For this review, take the finished solid that the model builds, in its own axes (mm). A direction names the side the tool comes from. Coordinates: 2 decimals unless noted, no trailing zeros. Order: outer loops, then holes, each group sorted by start corner. A loop starts at its lowest first (then second) coordinate and runs counter-clockwise, first axis right, second up. Notation, with made-up numbers: (-34.5, 6) -> (-6.5, 6) arc R17 ccw to (-6.5, 31) -> close; hole circle Ø11 at (38.25, -38). An arc over 180 degrees is marked (long way). Write item = value, one per line. Start each with the question number.
1) Insertion check: pin 1 Ø4.5 at (x, z) = (77, 50.13) entering from -Y; pin 2 Ø2 at (y, z) = (1, -73.5) entering from -X; pin 3 Ø1.1 at (y, z) = (4.5, -68) entering from -X; pin 4 Ø3 at (y, z) = (1, 76) entering from -X. Each pin has a flat end and moves straight along its axis. Give the tip position at first contact, or say it passes through.
2) Consider section D-D on x = 22. Give the boundary of the cut face in (y, z), and give its area (4 significant figures).
3) Machinability: for faces 4 (the face through (-1, 4, -74)), 5 (the face through (-78.984, 2.535, 51.65)), which of the approach directions +Z, -Z, +X, -X, +Y, -Y give a long, thin tool a straight path to every point of the face, cutting with its end or side? Answer none if there is none.
4) Consider section C-C on z = 70. Give the boundary of the cut face in (x, y).
5) Consider section A-A on x = -60. Give the boundary of the cut face in (y, z).
6) Consider section B-B on y = 2.1. State how many separate pieces and enclosed holes the cut face has, and give its area (3 significant figures).
7) Draft analysis for pull direction Z (two halves, no side actions). For faces 1 (the face through (75.016, 2.535, -22.35)), 2 (the face through (95.38, 2.46, -30.04)), 3 (the face through (-1, 5, -1)), state which applies: +Z half, -Z half, draft (parallel to the pull), parting line (faces both ways), or undercut.
8) Wall thickness on probe 1 along Z at (x, y) = (60, 3.4); probe 2 along X at (y, z) = (3.6, 52); probe 3 along Z at (x, y) = (77, 1.8): over which ranges is each line inside the solid? List them lowest first. Write a range as [from, to].
from build123d import *

# Parameters (mm, degrees)
SKETCH1_R           = 100
BOSS_EXTRUDE1_DEPTH = 5
SKETCH2_R           = 2.5
CUT_EXTRUDE1_DEPTH  = 10
SKETCH3_W           = 30
SKETCH3_H           = 30
CUT_EXTRUDE2_DEPTH  = 1


with BuildPart() as part:
    # Sketch1 → Boss-Extrude1 (new body)
    with BuildSketch(Plane(origin=(0, 0, 0), x_dir=(1, 0, 0), z_dir=(0, 1, 0))):
        Circle(SKETCH1_R)
    extrude(amount=BOSS_EXTRUDE1_DEPTH)

    # Sketch2 → Cut-Extrude1 (cut)
    with BuildSketch(Plane(origin=(0, 5, 0), x_dir=(1, 0, 0), z_dir=(0, 1, 0))):
        with Locations((-77, -50.128296411)):
            Circle(SKETCH2_R)
        with Locations((-77, 23.871703589)):
            Circle(SKETCH2_R)
        with Locations((-60, -50.128296411)):
            Circle(SKETCH2_R)
        with Locations((-60, 23.871703589)):
            Circle(SKETCH2_R)
        with Locations((60, 23.871703589)):
            Circle(SKETCH2_R)
        with Locations((60, -50.128296411)):
            Circle(SKETCH2_R)
        with Locations((77, 23.871703589)):
            Circle(SKETCH2_R)
        with Locations((77, -50.128296411)):
            Circle(SKETCH2_R)
    extrude(amount=-CUT_EXTRUDE1_DEPTH, mode=Mode.SUBTRACT)

    # Sketch3 → Cut-Extrude2 (cut)
    with BuildSketch(Plane(origin=(0, 5, 0), x_dir=(1, 0, 0), z_dir=(0, 1, 0))):
        with Locations((-0.508280415, 73.936051257)):
            Rectangle(SKETCH3_W, SKETCH3_H)
    extrude(amount=-CUT_EXTRUDE2_DEPTH, mode=Mode.SUBTRACT)


solid = part.part
Answer sheet:
q1.pin_1 = through
q1.pin_2 = -68.87
q1.pin_3 = -73.83
q1.pin_4 = -66.71
q2.outline = (0, -97.55) -> (5, -97.55) -> (5, 97.55) -> (0, 97.55) -> close
q2.area = 975.5 mm2
q3.face_4 = +Y
q3.face_5 = +Y, -Y
q4.outline = (-71.41, 0) -> (71.41, 0) -> (71.41, 5) -> (-71.41, 5) -> close
q5.outline = (0, -80) -> (5, -80) -> (5, -26.37) -> (0, -26.37) -> close; (0, -21.37) -> (5, -21.37) -> (5, 47.63) -> (0, 47.63) -> close; (0, 52.63) -> (5, 52.63) -> (5, 80) -> (0, 80) -> close
q6.separate_pieces = 1
q6.enclosed_holes = 8
q6.area = 31,300 mm2
q7.face_1 = undercut
q7.face_2 = parting line
q7.face_3 = draft
q8.probe_1 = [-80, -26.37], [-21.37, 47.63], [52.63, 80]
q8.probe_2 = [-85.42, -78.66], [-75.34, -61.66], [-58.34, 58.34], [61.66, 75.34], [78.66, 85.42]
q8.probe_3 = [-63.8, -26.37], [-21.37, 47.63], [52.63, 63.8]
